Read the model definition and answer for the solid it produces. Units are mm, in the model's axes. Face numbers are marked on the shaded views. A direction names the side the tool comes from. Coordinates: 2 decimals unless noted, no trailing zeros. Write each loop counter-clockwise with the first axis right and the second up, starting at its lowest first coordinate (ties: lowest second). Pieces come first, ordered by that corner, then holes. Notation, with made-up numbers: (62.25, -10) -> (109.25, -10) arc R16 ccw to (109.25, 17) -> close; hole circle Ø3 at (16, 2). An arc over 180 degrees is marked (long way). Return JSON: item names as keys, results as strings.
Autodesk Inventor part; units mm, degrees
ref_plane "YZ Plane" through (0, 0, 0) normal (1, 0, 0) x (0, 1, 0)
ref_plane "XZ Plane" through (0, 0, 0) normal (0, 1, 0) x (-1, 0, 0)
ref_plane "XY Plane" through (0, 0, 0) normal (0, 0, 1) x (1, 0, 0)
sketch "Sketch1" plane through (0, 0, 0) normal (0, 0, 1) x (1, 0, 0)
  line L0 (-82, -50) -> (82, -50)
  line L1 (82, -50) -> (82, 50)
  line L2 (82, 50) -> (-82, 50)
  line L3 (-82, 50) -> (-82, -50)
  line L4 (-82, -50) -> (82, 50) construction
  line L5 (82, -50) -> (-82, 50) construction
  point P0 (0, 0)
  dimension "d0" = 164
  dimension "d1" = 100
extrude "Extrusion1" add sketch "Sketch1" along normal mid plane 12
sketch "Sketch2" plane through (0, 0, 6) normal (0, 0, 1) x (1, 0, 0)
  line L0 (-82, 50) -> (-82, -50)
  line L1 (-82, -30) -> (-70, -30)
  line L2 (-70, -30) -> (-70, -10)
  line L3 (-70, -10) -> (-82, -10)
  line L4 (-82, -10) -> (-82, -30)
  line L5 (-82, -50) -> (82, -50)
  line L6 (-82, 10) -> (-70, 10)
  line L7 (-70, 10) -> (-70, 30)
  line L8 (-70, 30) -> (-82, 30)
  line L9 (-82, 30) -> (-82, 10)
  point P0 (0, 0)
  dimension "d4" = 12
  dimension "d5" = 20
  dimension "d6" = 20
  dimension "d7" = 20
  dimension "d8" = 20
extrude "Extrusion2" cut sketch "Sketch2" against normal through all
mirror "Mirror1" about plane through (0, 0, 0) normal (1, 0, 0) of "Extrusion2"
sketch "Sketch3" plane through (0, 0, 6) normal (0, 0, 1) x (1, 0, 0)
  line L0 (-40, -30) -> (40, -30)
  line L1 (50, -20) -> (50, 20)
  line L2 (40, 30) -> (-40, 30)
  line L3 (-50, 20) -> (-50, -20)
  line L4 (-50, -30) -> (50, 30) construction
  line L5 (50, -30) -> (-50, 30) construction
  arc A0 (-40, 30) -> (-50, 20) centre (-40, 20) ccw
  arc A1 (50, 20) -> (40, 30) centre (40, 20) ccw
  arc A2 (40, -30) -> (50, -20) centre (40, -20) ccw
  arc A3 (-50, -20) -> (-40, -30) centre (-40, -20) ccw
  point P0 (0, 0)
  dimension "d11" = 100
  dimension "d12" = 60
  dimension "d13" = 10
  dimension "d14" = 10
extrude "Extrusion3" cut sketch "Sketch3" against normal through all
sketch "Sketch5" plane through (0, 0, -6) normal (0, 0, -1) x (-1, 0, 0)
  line L0 (-40, 30) -> (40, 30)
  arc A0 (-40, 30) -> (-50, 20) centre (-40, 20) ccw
  line L1 (-50, -20) -> (-50, 20)
  arc A1 (-50, -20) -> (-40, -30) centre (-40, -20) ccw
  line L2 (40, -30) -> (-40, -30)
  arc A2 (40, -30) -> (50, -20) centre (40, -20) ccw
  line L3 (50, 20) -> (50, -20)
  arc A3 (50, 20) -> (40, 30) centre (40, 20) ccw
  line L4 (40, 38) -> (-40, 38)
  arc A4 (-40, 38) -> (-58, 20) centre (-40, 20) ccw
  line L5 (-58, 20) -> (-58, -20)
  arc A5 (-58, -20) -> (-40, -38) centre (-40, -20) ccw
  line L6 (-40, -38) -> (40, -38)
  arc A6 (40, -38) -> (58, -20) centre (40, -20) ccw
  line L7 (58, -20) -> (58, 20)
  arc A7 (58, 20) -> (40, 38) centre (40, 20) ccw
  point P0 (0, 0)
  dimension "d17" = 8
extrude "Extrusion4" cut sketch "Sketch5" against normal blind 3
properties part number "FRONT V2" material "Wood (Cherry)"
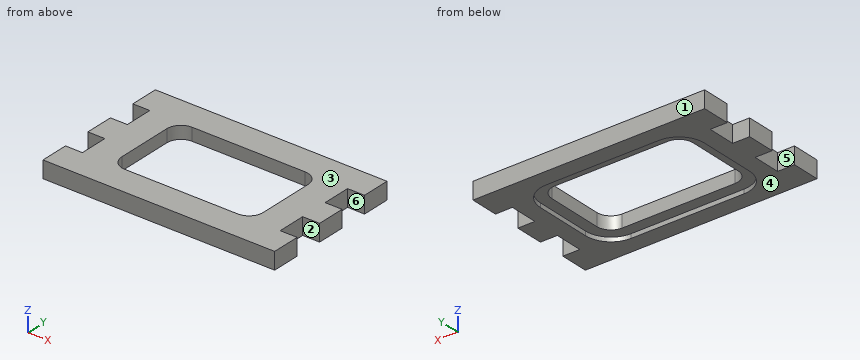
1. The part is cut by section C-C (y = 26.5). Determine the outline of the cut face in (x, z).
Taken from the geometry:
{"outline": "(-70, -6) -> (-56.79, -6) -> (-56.79, -3) -> (-47.6, -3) -> (-47.6, 6) -> (-70, 6) -> close; (47.6, -3) -> (56.79, -3) -> (56.79, -6) -> (70, -6) -> (70, 6) -> (47.6, 6) -> close"}
2. For a pull along Y with two mould halves and no side action, classify the marked faces 1, 2 and 3 as +Y half, -Y half, draft (parallel to the pull), parting line (faces both ways), or undercut.
Taken from the geometry:
{"face 1": "+Y half", "face 2": "undercut", "face 3": "draft"}
3. Consider L1, parallel to Y at x = -25.5, z = -3.75; L2, parallel to X at y = -10.5, z = -1; L3, parallel to X at y = 1, z = -0.75. Determine where each line is inside the solid, lowest interval first.
Taken from the geometry:
{"L1": "y = -50 to -38, 38 to 50", "L2": "x = -70 to -50, 50 to 70", "L3": "x = -82 to -50, 50 to 82"}
4. The part is cut by section D-D (x = -52.5). Determine the outline of the cut face in (y, z).
Taken from the geometry:
{"outline": "(-50, -6) -> (-32.95, -6) -> (-32.95, -3) -> (32.95, -3) -> (32.95, -6) -> (50, -6) -> (50, 6) -> (-50, 6) -> close"}
5. A tool of negligible diameter and unlimited length cuts with its end or side. For the marked faces 4, 5 and 6, from which of +Z, -Z, +X, -X, +Y, -Y can it reach the whole face along a straight path? Write none if from no direction.
Taken from the geometry:
{"face 4": "-Z, +X, -X, +Y, -Y", "face 5": "+Z, -Z, -X", "face 6": "+Z, -Z, +X"}
6. The part is cut by section A-A (x = -34.5). Determine the outline of the cut face in (y, z), then the cut area to 3 significant figures.
Taken from the geometry:
{"outline": "(-50, -6) -> (-38, -6) -> (-38, -3) -> (-30, -3) -> (-30, 6) -> (-50, 6) -> close; (30, -3) -> (38, -3) -> (38, -6) -> (50, -6) -> (50, 6) -> (30, 6) -> close", "area": "432 mm2"}
7. Flat-ended cylindrical pins translate along their axes: pin 1 Ø5 at (y, z) = (22.5, -0.5) entering from -X; pin 2 Ø3.5 at (y, z) = (-16, 2.5) entering from +X; pin 3 Ø6 at (x, y) = (21.5, 29.5) entering from -Z. Find the tip coordinate at first contact, or state that the pin passes through.
Taken from the geometry:
{"pin 1": "stops at x = -70", "pin 2": "stops at x = 70", "pin 3": "stops at z = -3"}
8. The part is cut by section B-B (z = 2.75). Determine the outline of the cut face in (x, y), then the cut area to 3 significant figures.
Taken from the geometry:
{"outline": "(-82, -50) -> (82, -50) -> (82, -30) -> (70, -30) -> (70, -10) -> (82, -10) -> (82, 10) -> (70, 10) -> (70, 30) -> (82, 30) -> (82, 50) -> (-82, 50) -> (-82, 30) -> (-70, 30) -> (-70, 10) -> (-82, 10) -> (-82, -10) -> (-70, -10) -> (-70, -30) -> (-82, -30) -> close; hole (-50, -20) arc R10 ccw to (-40, -30) -> (40, -30) arc R10 ccw to (50, -20) -> (50, 20) arc R10 ccw to (40, 30) -> (-40, 30) arc R10 ccw to (-50, 20) -> close", "area": "9,530 mm2"}
